```python
from build123d import *

# Parameters (mm, degrees)
F0_W        = 12.7
F0_H        = 12.7
F1_DEPTH    = 12.7
F2_W        = 6.35
F2_H        = 35.1087670878
F3_DEPTH    = 6.35
F4_R        = 1.27
F5_DEPTH    = 25.4
F6_T1_DEPTH = 36.2464301965


# Not quite as in the source:
# - a fillet or chamfer that OpenCascade refuses, or shapes differently, is made with other operations: its cross-section is extruded or revolved along the edge and cut away or added


with BuildPart() as f1:
    # F0 (on Top) → F1 (new body)
    with BuildSketch(Plane.XY):
        Rectangle(F0_W, F0_H)
    extrude(amount=F1_DEPTH)

    # F2 (on face) → F3 (cut)
    with BuildSketch(Plane(origin=(0, 0, 0), x_dir=(1, 0, 0), z_dir=(0, 0, -1))):
        Rectangle(F2_W, F2_H)
    extrude(amount=-F3_DEPTH, mode=Mode.SUBTRACT)

    # F4 (on face) → F5 (cut)
    with BuildSketch(Plane(origin=(-6.35, 0, 0), x_dir=(0, -1, 0), z_dir=(-1, 0, 0))):
        with Locations((0, 2.2022052582)):
            Circle(F4_R)
    extrude(amount=-F5_DEPTH, mode=Mode.SUBTRACT)

    # F6: fillet of radius 5.08 on 2 edges, made by hand

    # F6_s2 → F6_t1 (cut)
    with BuildSketch(Plane.XZ.offset(-18.1232150983)):
        with BuildLine():
            ThreePointArc((-3.175, 0), (-5.4821134838, 1.8694797079), (-6.35, 4.7092860393))
            Line((-6.35, 4.7092860393), (-6.35, 0))
            Line((-6.35, 0), (-3.175, 0))
        make_face()
        with BuildLine():
            ThreePointArc((3.175, 0), (5.4821134838, 1.8694797079), (6.35, 4.7092860393))
            Line((6.35, 4.7092860393), (6.35, 0))
            Line((6.35, 0), (3.175, 0))
        make_face()
    extrude(amount=F6_T1_DEPTH, mode=Mode.SUBTRACT)


solid = f1.part
```
Input: part model. Units: mm. Frame: model coordinates. A direction names the side the tool comes from. Give positions to 0.01 mm unless a question says otherwise; leave off trailing zeros. Order: outer loops, then holes, each group sorted by start corner. A loop starts at its lowest first (then second) coordinate and runs counter-clockwise, first axis right, second up. Notation, with made-up numbers: M 50.25,1 L 77.25,1 A13 ccw 77.25,13 Z; hole C -5.75,-28.75 d7. An arc over 180 degrees is marked long. One line per question, with ' | ' between items.
1) Draft query along Y for faces 1 (the face through (0, 0, 12.7)), 2 (the face through (0, -6.35, 8)), 3 (the face through (0, 6.35, 8)), 4 (the face through (-4.37, 0.17, 3.46)). Return one class per face: pulls with the +Y half, pulls with the -Y half, needs draft (parallel to the pull), parting line crosses it, or undercut.
Filled in:
face 1: needs draft | face 2: pulls with the -Y half | face 3: pulls with the +Y half | face 4: undercut
2) Section D-D on x = -2.5. Output: boundary loops of the cut face in (y, z).
Filled in:
outline: M -6.35,6.35 L 6.35,6.35 L 6.35,12.7 L -6.35,12.7 Z
3) Ray query, L1, parallel to X at y = -3.5, z = 6 (3 decimals); L2, parallel to Z at x = 4.2, y = 0; L3, parallel to Z at x = 4.75, y = 0. Return the intervals inside material, ascending.
Filled in:
L1: x = -6.35 to -3.175, 3.175 to 6.35 | L2: z = 0.56 to 0.93, 3.47 to 12.7 | L3: z = 3.47 to 12.7
4) Section A-A on z = 5.25. Output: boundary loops of the cut face in (x, y) (3 decimals).
Filled in:
outline: M -6.35,-6.35 L -3.175,-6.35 L -3.175,6.35 L -6.35,6.35 Z; M 3.175,-6.35 L 6.35,-6.35 L 6.35,6.35 L 3.175,6.35 Z
5) Access query for faces 5 (the face through (0, 0, 6.35)), 6 (the face through (4.33, 0.17, 3.46)). Directions: +Z, -Z, +X, -X, +Y, -Y. A direction counts if a zero-diameter tool reaches every point of the face in a straight line with its end or side. Return the directions, or none.
Filled in:
face 5: -Z, +Y, -Y | face 6: +X, -X
6) Section B-B on y = 0. Output: boundary loops of the cut face in (x, z) (3 decimals).
Filled in:
outline: M -6.35,4.709 A5.08 ccw -6.197,3.472 L -3.175,3.472 L -3.175,6.35 L 3.175,6.35 L 3.175,3.472 L 6.197,3.472 A5.08 ccw 6.35,4.709 L 6.35,12.7 L -6.35,12.7 Z; M -4.667,0.932 A5.08 ccw -3.175,0 L -3.175,0.932 Z; M 3.175,0 A5.08 ccw 4.667,0.932 L 3.175,0.932 Z
7) Section C-C on y = -3.25. Output: boundary loops of the cut face in (x, z) (3 decimals), and give its area (3 significant figures).
Filled in:
outline: M -6.35,4.709 A5.08 ccw -3.175,0 L -3.175,6.35 L 3.175,6.35 L 3.175,0 A5.08 ccw 6.35,4.709 L 6.35,12.7 L -6.35,12.7 Z | area: 113 mm2
8) Contact query for flat-ended pins moving along their axis: P1, Ø1.5, axis at y = 0, z = 2.2, coming from the -X side; P2, Ø1.9, axis at y = -1, z = 2.5, coming from the -X side; P3, Ø5, axis at x = 1.5, y = -1.5, coming from the -Z side; P4, Ø3, axis at y = 0, z = 2, coming from the +X side. Output: stop coordinate, or through.
Filled in:
P1: passes through | P2: stops at x = -6.19 | P3: stops at z = 0 | P4: stops at x = 6.2
